Read the model definition and answer for the solid it produces. Units are mm, in the model's axes. A direction names the side the tool comes from. Coordinates: 2 decimals unless noted, no trailing zeros. Loops run counter-clockwise (first coordinate to the right, second up) from the corner with the lowest first, then second, coordinate; pieces in that order, holes last.
Q1. Section A-A (x = 25) is taken. Give the vertices of the cut face in (y, z).
Q2. Flat-ended cylindrical pins translate along their axes: P1, Ø12, axis at x = 50, y = -5.5, coming from the +Z side; P2, Ø21, axis at x = 29, y = -25, coming from the +Z side; P3, Ø10, axis at x = 46, y = -22, coming from the +Z side; P4, Ø5, axis at x = 78.5, y = -8, coming from the +Z side. Find the tip coordinate at first contact, or state that the pin passes through.
Q3. Section B-B (z = 7) is taken. Give the vertices of the cut face in (x, y), then the cut area to 3 significant figures.
Q4. The mould has two halves that part along X. Classify faces 1 (the face through (55.091, -31.293, 4.563)), 2 (the face through (88.692, -35.834, 68.21)), 3 (the face through (9, -11, 4)), 4 (the face through (27.246, -20.348, 4.563)): pulls with the +X half, pulls with the -X half, needs draft (parallel to the pull), parting line crosses it, or undercut.
Q5. Section D-D (y = -38) is taken. Give the vertices of the cut face in (x, z).
Q6. Straight lines are drawn through the part: line 1 (X direction, y = -23, z = 3); line 2 (Y direction, x = 22, z = 6); line 3 (Z direction, x = 51.5, y = -23.5). For each, find the intervals that lie inside material, in ascending order.
Q7. Which of the six approach directions +Z, -Z, +X, -X, +Y, -Y give full straight-line access (tool end or side, diameter ignored) to faces 5 (the face through (83.955, -22.185, 66.673)), 6 (the face through (59, -15, 4)), 7 (the face through (92.833, -17.185, 70.522)), 8 (the face through (34, -22, 9))?
Q8. Section C-C (z = 45) is taken. Give the vertices of the cut face in (x, y).
from build123d import *

# Parameters (mm, degrees)
F1_DEPTH  = 9
F3_DEPTH  = 26
F5_DEPTH  = 35.001
F6_R      = 7
F7_DEPTH  = 9
F8_R      = 13
F9_R      = 5.5
F10_DEPTH = 9.001


with BuildPart() as f1:
    # F0 (on Front) → F1 (new body)
    with BuildSketch(Plane.XZ):
        Polygon((75.313708, 75.313708), (0, 0), (59, 0), (97.941125, 52.686292), align=None)
    extrude(amount=F1_DEPTH)

    # F2 (on face) → F3 (join)
    with BuildSketch(Plane.XZ.offset(9)):
        Polygon((0, 0), (59, 0), (59, 9), (9, 9), align=None)
    extrude(amount=F3_DEPTH)

    # F4 (on face) → F5 (cut, through all)
    with BuildSketch(Plane.XZ.offset(35)):
        Polygon((9, 9), (0, 0), (9, 0), align=None)
    extrude(amount=-F5_DEPTH, mode=Mode.SUBTRACT)

    # F6 (on face) → F7 (join)
    with BuildSketch(Plane(origin=(75.313708, 0, 75.313708), x_dir=(0.707107, 0, -0.707107), z_dir=(0.707107, 0, 0.707107))):
        with BuildLine():
            Line((32, 0), (0, 0))
            Line((0, 0), (0, -29))
            ThreePointArc((0, -29), (16, -45), (32, -29))
            Line((32, -29), (32, 0))
        make_face()
        with Locations((16, -29)):
            Circle(F6_R, mode=Mode.SUBTRACT)
    extrude(amount=F7_DEPTH)

    # F8
    f8_edges = [f1.edges().sort_by_distance(p)[0] for p in [
        (9, -35, 4.5),
        (59, -35, 4.5),
    ]]
    fillet(f8_edges, radius=F8_R)

    # F9 (on face) → F10 (cut, through all)
    with BuildSketch(Plane.XY.offset(9)):
        with Locations((22, -22)):
            Circle(F9_R)
        with Locations((46, -22)):
            Circle(F9_R)
    extrude(amount=-F10_DEPTH, mode=Mode.SUBTRACT)


solid = f1.part
Numbers:
1. outline: (-35, 0) - (-26.61, 0) - (-26.61, 9) - (-35, 9) - close; (-17.39, 0) - (0, 0) - (0, 25) - (-9, 25) - (-9, 9) - (-17.39, 9) - close
2. P1: stops at z = 56
2. P2: stops at z = 9
2. P3: passes through
2. P4: stops at z = 81
3. outline: (9, -22) arc R13 ccw to (22, -35) - (46, -35) arc R13 ccw to (59, -22) - (59, -9) - (64.17, -9) - (64.17, 0) - (9, 0) - close; hole circle Ø11 at (22, -22); hole circle Ø11 at (46, -22)
3. area: 1,530 mm2
4. face 1: pulls with the +X half
4. face 2: undercut
4. face 3: pulls with the -X half
4. face 4: undercut
5. outline: (77.27, 73.35) - (95.98, 54.65) - (102.35, 61.01) - (83.64, 79.72) - close
6. line 1: x = 9.04 to 16.59, 27.41 to 40.59, 51.41 to 58.96
6. line 2: y = -35 to -27.5, -16.5 to 0
6. line 3: z = 0 to 9
7. face 5: -Z, -X, -Y
7. face 6: +Z, -Z, +X, -Y
7. face 7: +Z, +X, +Y, -Y
7. face 8: +Z, +X, -X, -Y
8. outline: (45, -9) - (92.26, -9) - (92.26, 0) - (45, 0) - close
